from build123d import *

# Parameters (mm, degrees)
SKETCH1_R           = 8
BOSS_EXTRUDE1_DEPTH = 275
SKETCH2_R           = 6
BOSS_EXTRUDE2_DEPTH = 36
SKETCH3_R           = 5
BOSS_EXTRUDE3_DEPTH = 15
BOSS_EXTRUDE4_START = 9.15
SKETCH4_R           = 5
BOSS_EXTRUDE4_DEPTH = 9.15
SKETCH5_R           = 4.8
BOSS_EXTRUDE5_DEPTH = 1.15
BOSS_EXTRUDE6_START = 0.7
SKETCH7_R           = 5
BOSS_EXTRUDE6_DEPTH = 0.7


with BuildPart() as part:
    # Sketch1 → Boss-Extrude1 (new body)
    with BuildSketch(Plane.XY):
        Circle(SKETCH1_R)
    extrude(amount=-BOSS_EXTRUDE1_DEPTH)

    # Sketch2 → Boss-Extrude2 (add)
    with BuildSketch(Plane.XY):
        Circle(SKETCH2_R)
    extrude(amount=BOSS_EXTRUDE2_DEPTH)

    # Sketch3 → Boss-Extrude3 (add)
    with BuildSketch(Plane.XY.offset(36)):
        Circle(SKETCH3_R)
    extrude(amount=BOSS_EXTRUDE3_DEPTH)

    # Sketch4 → Boss-Extrude4 (add)
    with BuildSketch(Plane(origin=(0, 0, -275), x_dir=(-1, 0, 0), z_dir=(0, 0, -1)).offset(BOSS_EXTRUDE4_START)):
        with Locations(Location((0, 0, 0), (0, 0, 180))):
            Circle(SKETCH4_R)
    extrude(amount=-BOSS_EXTRUDE4_DEPTH)

    # Sketch5 → Boss-Extrude5 (add)
    with BuildSketch(Plane(origin=(0, 0, -284.15), x_dir=(-1, 0, 0), z_dir=(0, 0, -1))):
        Circle(SKETCH5_R)
    extrude(amount=BOSS_EXTRUDE5_DEPTH)

    # Sketch7 → Boss-Extrude6 (add)
    with BuildSketch(Plane(origin=(0, 0, -285.3), x_dir=(-1, 0, 0), z_dir=(0, 0, -1)).offset(BOSS_EXTRUDE6_START)):
        with Locations(Location((0, 0, 0), (0, 0, 180))):
            Circle(SKETCH7_R)
    extrude(amount=-BOSS_EXTRUDE6_DEPTH)


solid = part.part
Check sheet for the modelled part. Datum: model origin and axes. Units: mm. A direction names the side the tool comes from. Round coordinates to 2 decimals unless told otherwise and drop trailing zeros. Loops run counter-clockwise (first coordinate to the right, second up) from the corner with the lowest first, then second, coordinate; pieces in that order, holes last.
1. Set-up check for faces 1 (the flat face through (0, 0, 51)), 2 (the cylindrical face through (-4.995, -0.22, -285.655)), 3 (the flat face through (-2, 6, 0)): record each of +Z, -Z, +X, -X, +Y, -Y from which the full face is reachable in a straight line by a thin tool's end or side.
2. Sectioned sample at A-A on x = 0. Record the boundary of the cut face in (y, z).
3. Scan lines: probe 1 along Y at (x, z) = (1, -82.5); probe 2 along X at (y, z) = (0.75, 21); probe 3 along Z at (x, y) = (5.25, 4.75). Record each from-to range of solid material in increasing order.
4. Sectioned sample at C-C on z = -146.5. Record the boundary of the cut face in (x, y), and give its area (3 significant figures).
5. Gauge pin test, flat ends, axial feed: pin 1 Ø6 at (x, z) = (1, -138) entering from +Y; pin 2 Ø3 at (x, z) = (2, -178.5) entering from -Y; pin 3 Ø4 at (y, z) = (5, -137) entering from -X; pin 4 Ø2 at (x, z) = (-3, -162) entering from +Y. Record the tip position at first contact, or that the pin passes through.
Recorded:
1. face 1: +Z, +X, -X, +Y, -Y
1. face 2: -Z
1. face 3: +Z
2. outline: (-8, -275) - (-5, -275) - (-5, -284.15) - (-4.8, -284.15) - (-4.8, -285.3) - (-5, -285.3) - (-5, -286) - (5, -286) - (5, -285.3) - (4.8, -285.3) - (4.8, -284.15) - (5, -284.15) - (5, -275) - (8, -275) - (8, 0) - (6, 0) - (6, 36) - (5, 36) - (5, 51) - (-5, 51) - (-5, 36) - (-6, 36) - (-6, 0) - (-8, 0) - close
3. probe 1: y = -7.94 to 7.94
3. probe 2: x = -5.95 to 5.95
3. probe 3: z = -275 to 0
4. outline: circle Ø16 at (0, 0)
4. area: 201 mm2
5. pin 1: stops at y = 8
5. pin 2: stops at y = -7.98
5. pin 3: stops at x = -7.42
5. pin 4: stops at y = 7.75
